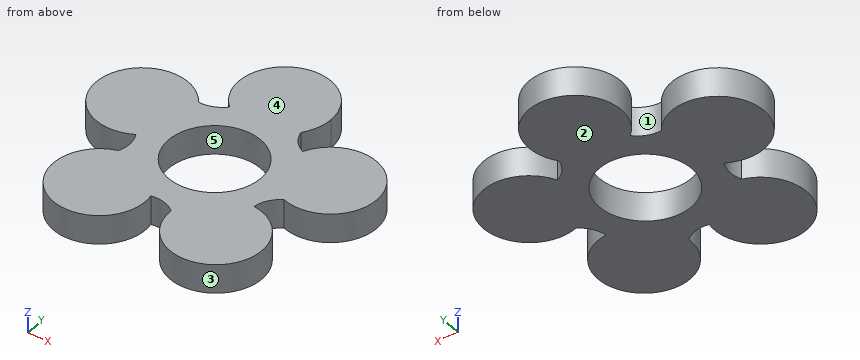
from build123d import *

# Parameters (mm, degrees)
F0_R     = 11.15
F1_DEPTH = 7


with BuildPart() as f1:
    # F0 (on Top) → F1 (new body)
    with BuildSketch(Plane.XY):
        with BuildLine():
            ThreePointArc((12.720798, 12.13026), (10.156571, 14.156134), (8.770986, 17.115793))
            ThreePointArc((8.770986, 17.115793), (10.538477, 20.358159), (11.15, 24))
            ThreePointArc((11.15, 24), (-4.445213, 34.225585), (-7.60562, 15.846654))
            ThreePointArc((-7.60562, 15.846654), (-10.324731, 14.03396), (-13.567703, 13.630774))
            ThreePointArc((-13.567703, 13.630774), (-33.664157, 10.032303), (-17.421329, -2.336489))
            ThreePointArc((-17.421329, -2.336489), (-16.537606, -5.48267), (-17.156287, -8.691511))
            ThreePointArc((-17.156287, -8.691511), (-19.944084, -28.916363), (-3.161354, -17.290683))
            ThreePointArc((-3.161354, -17.290683), (0.103928, -17.422436), (2.964534, -19.002424))
            ThreePointArc((2.964534, -19.002424), (21.338035, -27.903599), (15.467505, -8.349741))
            ThreePointArc((15.467505, -8.349741), (16.601837, -5.284987), (18.98847, -3.052632))
            ThreePointArc((18.98847, -3.052632), (33.131715, 11.670991), (12.720798, 12.13026))
        make_face()
        Circle(F0_R, mode=Mode.SUBTRACT)
    extrude(amount=F1_DEPTH)


solid = f1.part
CAD build for the part. Positions are in the model's coordinates, mm. Face numbers are marked on the shaded views. A direction names the side the tool comes from. Round coordinates to 2 decimals unless told otherwise and drop trailing zeros. Loops run counter-clockwise (first coordinate to the right, second up) from the corner with the lowest first, then second, coordinate; pieces in that order, holes last. Notation, with made-up numbers: (40, -1) - (79, -1) arc R23 cw to (79, 8) - close; hole circle Ø7 at (4, -39). An arc over 180 degrees is marked (long way). Put each result on its own line as item: value.
1. Slice it at A-A on y = 8. List the corners of the cut face in (x, z).
Geometry check:
outline: (-33.96, 0) - (-7.77, 0) - (-7.77, 7) - (-33.96, 7) - close; (7.77, 0) - (33.96, 0) - (33.96, 7) - (7.77, 7) - close
2. Slice it at C-C on z = 5. List the corners of the cut face in (x, y).
Geometry check:
outline: (-17.42, -2.34) arc R7.1 cw to (-17.16, -8.69) arc R11.15 ccw (long way) to (-3.16, -17.29) arc R7.1 cw to (2.96, -19) arc R11.15 ccw (long way) to (15.47, -8.35) arc R7.1 cw to (18.99, -3.05) arc R11.15 ccw (long way) to (12.72, 12.13) arc R7.1 cw to (8.77, 17.12) arc R11.15 ccw to (11.15, 24) arc R11.15 ccw (long way) to (-7.61, 15.85) arc R7.1 cw to (-13.57, 13.63) arc R11.15 ccw (long way) to start; hole circle Ø22.3 at (0, 0)
3. Wall check: line 1 (X direction, y = 16.5, z = 5.25); line 2 (X direction, y = -18, z = 5.5); line 3 (X direction, y = 4, z = 6). Give the ranges that are in metal, low to high.
Geometry check:
line 1: -29.29 to -16.36, -8.25 to 8.93, 16.36 to 29.29
line 2: -25.17 to -3.05, 1.54 to 25.17
line 3: -33.44 to -10.41, 10.41 to 33.44
4. Pin check, flat tips, straight feed: P1, Ø1.5, axis at x = -0.5, z = 5.5, coming from the -Y side; P2, Ø1, axis at x = 26.5, z = 4.5, coming from the -Y side; P3, Ø1, axis at y = 20, z = 2.5, coming from the +X side. Stop position of each tip, or through.
Geometry check:
P1: y = -17.46
P2: y = -3.27
P3: x = 10.59
5. 3-axis set-ups, long thin cutter, end or side, ignore diameter. For the marked faces 1 and 2: which of +Z, -Z, +X, -X, +Y, -Y reach the whole face in a straight line?
Geometry check:
face 1: +Z, -Z
face 2: -Z, +X, -X, +Y, -Y
6. Slice it at B-B on x = 0. List the corners of the cut face in (y, z).
Geometry check:
outline: (-17.39, 0) - (-11.15, 0) - (-11.15, 7) - (-17.39, 7) - close; (11.15, 0) - (35.15, 0) - (35.15, 7) - (11.15, 7) - close
7. Slice it at D-D on x = 29. List the corners of the cut face in (y, z), and give its area (3 significant figures).
Geometry check:
outline: (-1.87, 0) - (16.7, 0) - (16.7, 7) - (-1.87, 7) - close
area: 130 mm²
8. Two-plate mould, pull along Y, no slides. Class the marked faces 3, 4 and 5: released by +Y, released by -Y, zero draft, split by the parting line, or undercut.
Geometry check:
face 3: undercut
face 4: zero draft
face 5: undercut
